from build123d import *

# Parameters (mm, degrees)
F1_DEPTH = 19.4
F2_DEPTH = 1.2
F3_W     = 25
F3_H     = 7.2
F4_DEPTH = 1.2
F5_W     = 16.95
F5_H     = 7.1
F6_DEPTH = 9
F7_W     = 2.4
F7_H     = 1.2
F8_ANGLE = 180


with BuildPart() as f1:
    # F0 (on Right) → F1 (new body)
    with BuildSketch(Plane.YZ):
        Polygon((-8.6684125125, 6.8394026556), (-18.6684125125, 6.8394026556), (-18.6684125125, -2.3605973444), (-8.6684125125, -2.3605973444), (-8.6684125125, -1.3605973444), (-8.6684125125, 2.2394026556), (-8.6684125125, 5.8394026556), align=None)
    extrude(amount=F1_DEPTH)

    # F0 (on Right) → F2 (join)
    with BuildSketch(Plane.YZ):
        Polygon((-8.6684125125, 6.8394026556), (-18.6684125125, 6.8394026556), (-18.6684125125, -2.3605973444), (-8.6684125125, -2.3605973444), (-8.6684125125, -1.3605973444), (-8.6684125125, 2.2394026556), (-8.6684125125, 5.8394026556), align=None)
        Polygon((16.3315874875, 5.8394026556), (-8.6684125125, 5.8394026556), (-8.6684125125, 2.2394026556), (-8.6684125125, -1.3605973444), (16.3315874875, -1.3605973444), align=None)
        with BuildLine():
            ThreePointArc((1.3315874875, 1.2072022274), (0.6686982275, 2.2757759463), (1.4412960947, 3.267927396))
            Line((1.4412960947, 3.267927396), (11.4315874875, 3.3328592428))
            ThreePointArc((11.4315874875, 3.3328592428), (12.3394869948, 2.2497630325), (11.4315874875, 1.1666668222))
            Line((11.4315874875, 1.1666668222), (1.3315874875, 1.2072022274))
        make_face(mode=Mode.SUBTRACT)
    extrude(amount=F2_DEPTH)

    # F3 (on face) → F4 (join)
    with BuildSketch(Plane.YZ.offset(19.4)):
        with Locations((3.8315874875, 2.2394026556)):
            Rectangle(F3_W, F3_H)
        with BuildLine():
            ThreePointArc((1.3613110944, 1.1667440413), (0.6984218344, 2.2353177601), (1.4710197016, 3.2274692099))
            Line((1.4710197016, 3.2274692099), (11.4315874875, 3.292145016))
            Line((11.4315874875, 3.292145016), (11.4315874875, 3.2924010566))
            ThreePointArc((11.4315874875, 3.2924010566), (11.4322813424, 3.2922777636), (11.4329751181, 3.2921540261))
            ThreePointArc((11.4329751181, 3.2921540261), (12.3394869633, 2.2090418078), (11.4324572213, 1.1263632544))
            ThreePointArc((11.4324572213, 1.1263632544), (11.4320223699, 1.1262858579), (11.4315874875, 1.1262086361))
            Line((11.4315874875, 1.1262086361), (11.4315874875, 1.1263667416))
            Line((11.4315874875, 1.1263667416), (1.3613110944, 1.1667440413))
        make_face(mode=Mode.SUBTRACT)
    extrude(amount=-F4_DEPTH)

    # F5 (on face) → F6 (cut)
    with BuildSketch(Plane(origin=(0, -8.6684125125, 0), x_dir=(-1, 0, 0), z_dir=(0, 1, 0))):
        with Locations((-9.725, 2.2394026556)):
            Rectangle(F5_W, F5_H)
    extrude(amount=-F6_DEPTH, mode=Mode.SUBTRACT)

    # F7 (on face) → F8 (revolve)
    with BuildSketch(Plane.YZ.offset(19.4)):
        with Locations((-11.550808993, 2.5371138187)):
            Rectangle(F7_W, F7_H)
    revolve(axis=Axis((19.4, -13.350808993, 2.5371138187), (0, 0, -1)), revolution_arc=F8_ANGLE)


solid = f1.part
Work out the finished part from the listing and answer in its coordinate system (mm). A direction names the side the tool comes from. Round coordinates to 2 decimals unless told otherwise and drop trailing zeros. Order: outer loops, then holes, each group sorted by start corner. A loop starts at its lowest first (then second) coordinate and runs counter-clockwise, first axis right, second up. Notation, with made-up numbers: M -12,32 L 18,32 A31 cw 18,70 Z; hole C 53,20 d6. An arc over 180 degrees is marked long. Put each result on its own line as item: value. Start each with the question number.
Q1. Straight lines are drawn through the part: L1, parallel to X at y = 1.5, z = 4; L2, parallel to Z at x = 3.75, y = -10.5; L3, parallel to Y at x = 6.5, z = 6. For each, find the intervals that lie inside material, in ascending order. Write a range as [from, to].
Q2. Section D-D, the plane x = 11.75 is taken. Write down the section's boundary in (y, z), and give its area (3 significant figures).
Q3. For a pull along Z with two mould halves and no side action, classify faces 1 (the flat face through (1.2, 4, 4)), 2 (the flat face through (1, 4, 5.839)), 3 (the flat face through (10, -13, 5.789)), 4 (the cylindrical face through (0.592, 0.668, 2.257)) as pulls with the +Z half, pulls with the -Z half, needs draft (parallel to the pull), parting line crosses it, or undercut.
Q4. Section A-A, the plane y = 10 is taken. Write down the section's boundary in (x, z), and give its area (3 significant figures).
Q5. Section C-C, the plane y = -9.5 is taken. Write down the section's boundary in (x, z).
Q6. Flat-ended cylindrical pins translate along their axes: pin 1 (2 mm diameter, centred on y = 6, z = 2.5, fed in from +X); pin 2 (1 mm diameter, centred on x = 0.5, y = 3.5, fed in from -Z); pin 3 (1.3 mm diameter, centred on x = 18.5, y = 3, fed in from +Z); pin 4 (2 mm diameter, centred on x = 2.5, y = -3, fed in from +Z). Find the tip coordinate at first contact, or state that the pin passes through.
Q7. A tool of negligible diameter and unlimited length cuts with its end or side. For faces 5 (the flat face through (19, 4, 5.839)), 6 (the flat face through (19, 4, -1.361)), 7 (the flat face through (10, -17.668, 2)), from which of +Z, -Z, +X, -X, +Y, -Y can it reach the whole face along a straight path? Write none if from no direction.
Q8. Section B-B, the plane z = 4.5 is taken. Write down the section's boundary in (x, y).
Findings below:
1. L1: x = [0, 1.2], [18.2, 19.4]
1. L2: z = [-2.36, -1.31], [5.79, 6.84]
1. L3: y = [-18.67, -8.67]
2. outline: M -18.67,-2.36 L -8.67,-2.36 L -8.67,-1.31 L -17.67,-1.31 L -17.67,5.79 L -8.67,5.79 L -8.67,6.84 L -18.67,6.84 Z
2. area: 28.1 mm^2
3. face 1: needs draft
3. face 2: pulls with the +Z half
3. face 3: undercut
3. face 4: undercut
4. outline: M 0,-1.36 L 1.2,-1.36 L 1.2,1.17 L 0,1.17 Z; M 0,3.32 L 1.2,3.32 L 1.2,5.84 L 0,5.84 Z; M 18.2,-1.36 L 19.4,-1.36 L 19.4,1.13 L 18.2,1.13 Z; M 18.2,3.28 L 19.4,3.28 L 19.4,5.84 L 18.2,5.84 Z
4. area: 12.1 mm^2
5. outline: M 0,-2.36 L 19.4,-2.36 L 19.4,6.84 L 0,6.84 Z; hole M 1.25,-1.31 L 18.2,-1.31 L 18.2,5.79 L 1.25,5.79 Z
6. pin 1: stops at x = 19.4
6. pin 2: stops at z = -1.36
6. pin 3: stops at z = 5.84
6. pin 4: passes through
7. face 5: +Z, +X, -X, +Y
7. face 6: -Z, +X, -X, +Y
7. face 7: +Y
8. outline: M 0,-18.67 L 19.4,-18.67 L 19.4,16.33 L 18.2,16.33 L 18.2,-17.67 L 1.25,-17.67 L 1.25,-8.67 L 1.2,-8.67 L 1.2,16.33 L 0,16.33 Z
